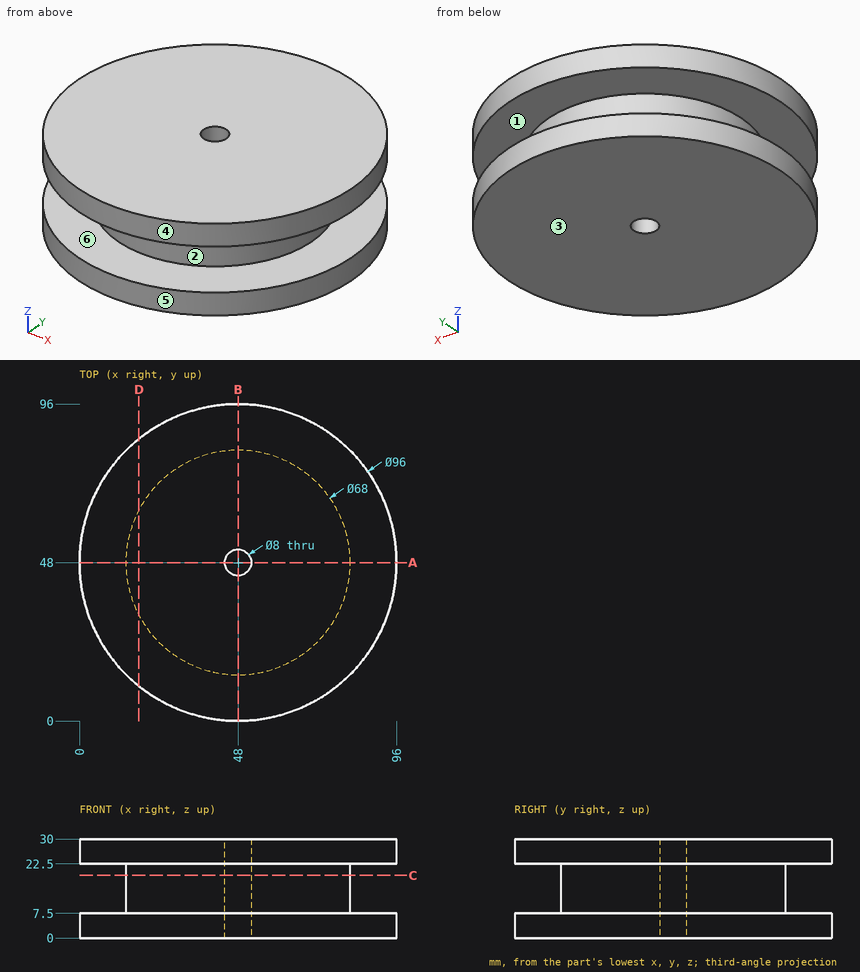
Here's the drawing with two shaded views (mm, measured from the low corner). I have some questions. A direction names the side the tool comes from. Round coordinates to 2 decimals unless told otherwise and drop trailing zeros. Loops run counter-clockwise (first coordinate to the right, second up) from the corner with the lowest first, then second, coordinate; pieces in that order, holes last. Notation, with made-up numbers: M 37.25,36.5 L 70.25,36.5 A18 ccw 70.25,47.5 Z; hole C -1,57 d2. An arc over 180 degrees is marked long. Answer as a JSON object with one key per item and string values. Group by question number.
Q1. We'd pull the mould along Z, two halves only. Please class the marked faces 1, 2, 3 and 4: +Z half, -Z half, draft (parallel to the pull), parting line (faces both ways), or undercut.
Q2. Imagine slicing it at D-D, the plane x = 18. Please give me the cut outline in (y, z).
Q3. Imagine slicing it at A-A, the plane y = 48. Please give me the cut outline in (x, z).
Q4. Imagine slicing it at C-C, the plane z = 19. Please give me the cut outline in (x, y), then the cut area to 3 significant figures.
Q5. Please list where these lines run through material, in increasing order: L1, parallel to Y at x = 48, z = 13.25; L2, parallel to Z at x = 31, y = 90.5; L3, parallel to Y at x = 48, z = 23.5.
Q6. On a 3-axis mill with a long thin cutter (end or side, diameter ignored), from which of +Z, -Z, +X, -X, +Y, -Y can I reach the whole of each face in a straight line? I mean the marked faces 5 and 6. Say none if no direction works.
Q7. Will these pins go through, and if not, where does the flat tip stop? pin 1 (6 mm diameter, centred on x = 66, z = 13, fed in from -Y); pin 2 (12 mm diameter, centred on x = 19.5, z = 6, fed in from -Y); pin 3 (2 mm diameter, centred on x = 68, z = 14, fed in from +Y).
Findings:
{
 "1": {"face 1": "undercut", "face 2": "undercut", "face 3": "-Z half", "face 4": "draft"},
 "2": {"outline": "M 10.53,0 L 85.47,0 L 85.47,7.5 L 64,7.5 L 64,22.5 L 85.47,22.5 L 85.47,30 L 10.53,30 L 10.53,22.5 L 32,22.5 L 32,7.5 L 10.53,7.5 Z"},
 "3": {"outline": "M 0,0 L 44,0 L 44,30 L 0,30 L 0,22.5 L 14,22.5 L 14,7.5 L 0,7.5 Z; M 52,0 L 96,0 L 96,7.5 L 82,7.5 L 82,22.5 L 96,22.5 L 96,30 L 52,30 Z"},
 "4": {"outline": "C 48,48 d68; hole C 48,48 d8", "area": "3,580 mm2"},
 "5": {"L1": "y = 14 to 44, 52 to 82", "L2": "z = 0 to 7.5, 22.5 to 30", "L3": "y = 0 to 44, 52 to 96"},
 "6": {"face 5": "+Z, -Z", "face 6": "none"},
 "7": {"pin 1": "stops at y = 17.49", "pin 2": "stops at y = 5.6", "pin 3": "stops at y = 76.2"}
}
